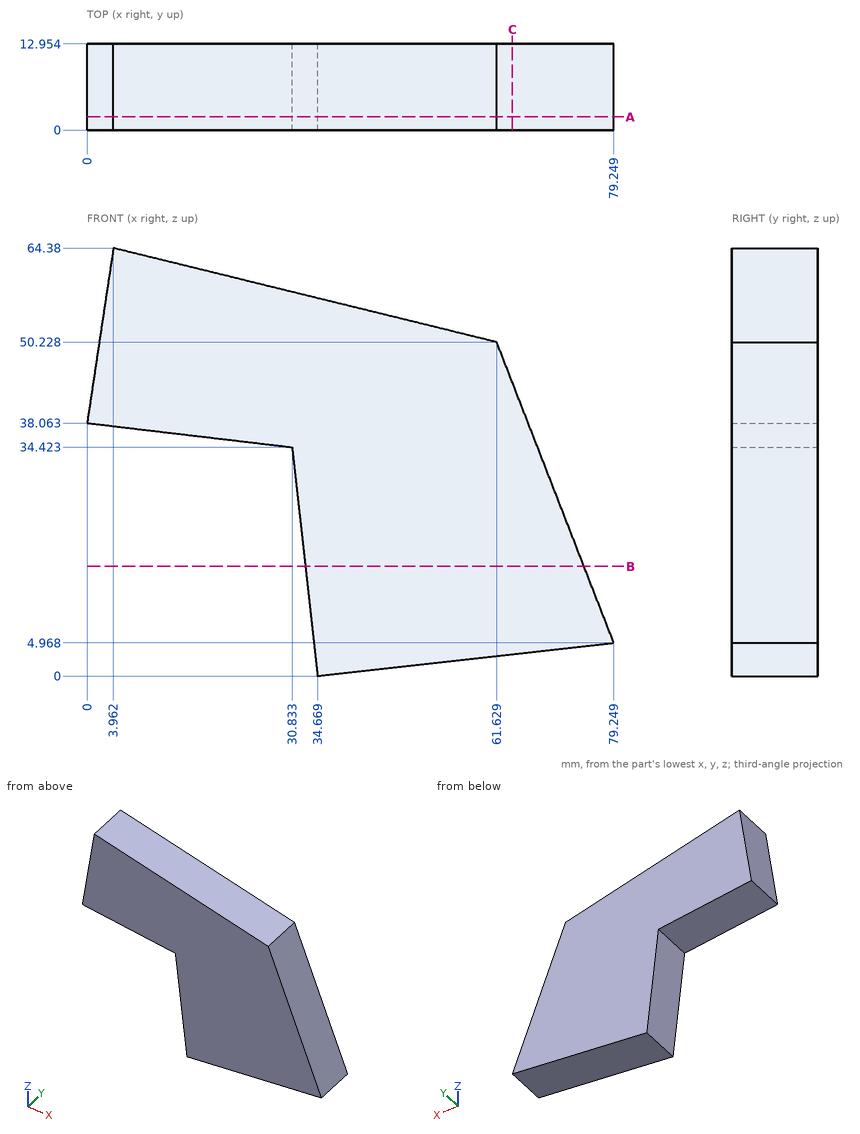
Part print with two shaded views. Sizes in mm from the minimum x, y, z corner. Give positions to 0.01 mm unless a question says otherwise; leave off trailing zeros. Order: outer loops, then holes, each group sorted by start corner. A loop starts at its lowest first (then second) coordinate and runs counter-clockwise, first axis right, second up. Notation, with made-up numbers: (24, 26) - (48, 26) arc R31 ccw to (48, 64) - close; hole circle Ø2 at (77, -14). An arc over 180 degrees is marked (long way). Write each question's results on one line, items separated by ' | '.
1. Saw through at C-C on x = 64. List the corners of the cut face in (y, z).
Calculated:
outline: (0, 3.27) - (12.95, 3.27) - (12.95, 44.14) - (0, 44.14) - close
2. Saw through at B-B on z = 16.5. List the corners of the cut face in (x, y).
Calculated:
outline: (32.83, 0) - (74.76, 0) - (74.76, 12.95) - (32.83, 12.95) - close
3. Saw through at A-A on y = 2. List the corners of the cut face in (x, z).
Calculated:
outline: (0, 38.06) - (30.83, 34.42) - (34.67, 0) - (79.25, 4.97) - (61.63, 50.23) - (3.96, 64.38) - close
4. Probe L1, parallel to Z at x = 6, y = 5.5 (1 decimal); L2, parallel to X at y = 12.5, z = 49 (1 decimal); L3, parallel to Z at x = 30, y = 4. List the from-to ranges inside material, lowest first. Write a range as from..to.
Calculated:
L1: z = 37.4..63.9 | L2: x = 1.6..62.1 | L3: z = 34.52..57.99
5. Pin check, flat tips, straight feed: pin 1 (4 mm diameter, centred on x = 10.5, y = 5, fed in from +Z); pin 2 (2 mm diameter, centred on x = 26, y = 5, fed in from +Z); pin 3 (2 mm diameter, centred on y = 11, z = 14.5, fed in from +X). Stop position of each tip, or through.
Calculated:
pin 1: stops at z = 63.27 | pin 2: stops at z = 59.22 | pin 3: stops at x = 75.93
